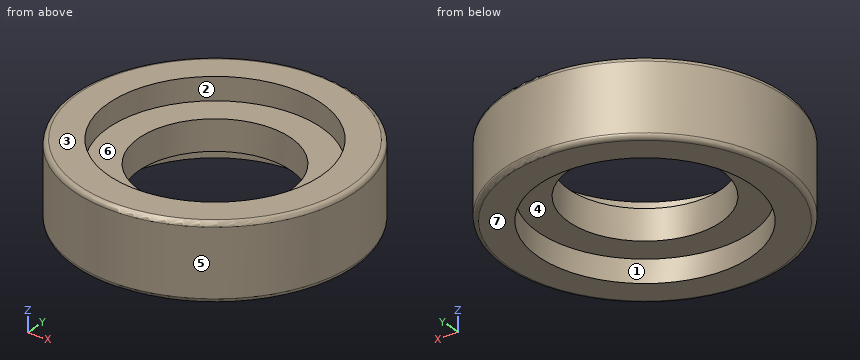
```python
from build123d import *

# Parameters (mm, degrees)
F0_R     = 9.25
F0_R_2   = 7
F1_DEPTH = 2.5
F0_R_3   = 5
F2_DEPTH = 1
F3_R     = 0.3


with BuildPart() as f1:
    # F0 (on Top) → F1 (new body, symmetric)
    with BuildSketch(Plane.XY):
        Circle(F0_R)
        Circle(F0_R_2, mode=Mode.SUBTRACT)
    extrude(amount=F1_DEPTH, both=True)

    # F0 (on Top) → F2 (join, symmetric)
    with BuildSketch(Plane.XY):
        Circle(F0_R_2)
        Circle(F0_R_3, mode=Mode.SUBTRACT)
    extrude(amount=F2_DEPTH, both=True)

    # F3
    f3_edges = [f1.edges().sort_by_distance(p)[0] for p in [
        (-9.25, 0, 2.5),
        (-9.25, 0, -2.5),
    ]]
    fillet(f3_edges, radius=F3_R)


solid = f1.part
```
Check sheet for the modelled part. Datum: model origin and axes. Units: mm. Face numbers are marked on the shaded views. A direction names the side the tool comes from. Give positions to 0.01 mm unless a question says otherwise; leave off trailing zeros. Write each loop counter-clockwise with the first axis right and the second up, starting at its lowest first coordinate (ties: lowest second). Pieces come first, ordered by that corner, then holes.
Item 1: Cross-section at A-A (y = 0). Enter the section's corners in (x, z), and give its area (3 significant figures).
Item 2: Access from +Z, -Z, +X, -X, +Y, -Y to the whole of each face (thin tool, end or side, straight path). Record for the marked faces 1, 2 and 3.
Item 3: Cross-section at C-C (z = 0.7). Enter the section's corners in (x, y).
Item 4: Scan lines: L1, parallel to Y at x = 0, z = -2.05; L2, parallel to X at y = -4.5, z = 1.95; L3, parallel to Z at x = 4.25, y = 3.5. Record each from-to range of solid material in increasing order.
Item 5: Cross-section at D-D (z = -1.3). Enter the section's corners in (x, y).
Item 6: Gauge pin test, flat ends, axial feed: pin 1 (3 mm diameter, centred on y = -3, z = -0.5, fed in from +X); pin 2 (2 mm diameter, centred on x = 7, z = -1, fed in from -Y); pin 3 (7 mm diameter, centred on x = -1.5, y = 2.5, fed in from +Z). Record the tip position at first contact, or that the pin passes through.
Item 7: Draft check along Y on the marked faces 4, 5, 6 and 7. Enter one of: released by +Y, released by -Y, zero draft, split by the parting line, or undercut.
Report:
1. outline: (-9.25, -2.2) arc R0.3 ccw to (-8.95, -2.5) - (-7, -2.5) - (-7, -1) - (-5, -1) - (-5, 1) - (-7, 1) - (-7, 2.5) - (-8.95, 2.5) arc R0.3 ccw to (-9.25, 2.2) - close; (5, -1) - (7, -1) - (7, -2.5) - (8.95, -2.5) arc R0.3 ccw to (9.25, -2.2) - (9.25, 2.2) arc R0.3 ccw to (8.95, 2.5) - (7, 2.5) - (7, 1) - (5, 1) - close
1. area: 30.4 mm2
2. face 1: -Z
2. face 2: +Z
2. face 3: +Z, +X, -X, +Y, -Y
3. outline: circle Ø18.5 at (0, 0); hole circle Ø10 at (0, 0)
4. L1: y = -9.25 to -7, 7 to 9.25
4. L2: x = -8.08 to -5.36, 5.36 to 8.08
4. L3: z = -1 to 1
5. outline: circle Ø18.5 at (0, 0); hole circle Ø14 at (0, 0)
6. pin 1: stops at x = 9.13
6. pin 2: stops at y = -7.04
6. pin 3: stops at z = 1
7. face 4: undercut
7. face 5: split by the parting line
7. face 6: undercut
7. face 7: zero draft
